Geometry: final body of the model. Coordinates: model frame, mm. A direction names the side the tool comes from. Give positions to 0.01 mm unless a question says otherwise; leave off trailing zeros. Write each loop counter-clockwise with the first axis right and the second up, starting at its lowest first coordinate (ties: lowest second). Pieces come first, ordered by that corner, then holes. Notation, with made-up numbers: (47, 66) -> (83, 66) arc R18 ccw to (83, 75) -> close; hole circle Ø8 at (-38, 39.5). An arc over 180 degrees is marked (long way). Answer in a Markdown table with one row per item. Add a question column.
Item 1: First-contact query: P1, Ø0.7, axis at y = 26, z = 2.5, coming from the +X side; P2, Ø2, axis at y = -28, z = 2, coming from the -X side; P3, Ø2, axis at y = -103.5, z = 1, coming from the -X side. Flat tips, straight axial feed; report the tip coordinate or a pass-through.
Item 2: Access query for faces 4 (the flat face through (-12.56, -102, 2)), 5 (the flat face through (5, -38.987, 2)), 6 (the flat face through (39.56, -102, 2)), 7 (the flat face through (-7, -60.137, 2)), 8 (the flat face through (2, -34.637, 2)). Directions: +Z, -Z, +X, -X, +Y, -Y. A direction counts if a zero-diameter tool reaches every point of the face in a straight line with its end or side. Return the directions, or none.
Item 3: Draft query along X for faces 1 (the flat face through (-4, -6, 2)), 2 (the flat face through (-2, -10.137, 2)), 3 (the cylindrical face through (14.54, -8.13, 1.97)). Return one class per face: +X half, -X half, draft (parallel to the pull), parting line (faces both ways), or undercut.
Item 4: Section query C-C on x = 13.5. Output: boundary loops of the cut face in (y, z), plus the area to 3 significant figures.
Item 5: Material intervals for probe 1 along Y at (x, z) = (21.5, 1); probe 2 along Y at (x, z) = (13.5, 3.1); probe 3 along X at (y, z) = (-38, 2.85), sorted ascending. Write a range as from..to.
Item 6: Section query A-A on x = -15.56. Output: boundary loops of the cut face in (y, z), plus the area to 3 significant figures.
Item 7: Section query B-B on x = 1.5. Output: boundary loops of the cut face in (y, z).
Item 8: Section query D-D on x = 42.56. Output: boundary loops of the cut face in (y, z).
```python
from build123d import *

# Parameters (mm, degrees)
SKETCH_1_R      = 2.25
SKETCH_1_R_2    = 2
SKETCH_1_R_3    = 4.1
SKETCH_1_R_4    = 1.5
EXTRUDE_1_DEPTH = 4


with BuildPart() as part:
    # 草图1 → 凸台-拉伸1 (new body)
    with BuildSketch(Plane.XY):
        with BuildLine():
            Line((0, -10.136956522), (-4, -10.136956522))
            Line((-4, -10.136956522), (-4, -2.136956522))
            Line((-4, -2.136956522), (0, -2.136956522))
            Line((0, -2.136956522), (0, 22.363043478))
            Line((0, 22.363043478), (4, 22.363043478))
            Line((4, 22.363043478), (4, 21.013043478))
            Line((4, 21.013043478), (6.6, 21.013043478))
            Line((6.6, 21.013043478), (6.6, 22.363043478))
            Line((6.6, 22.363043478), (8.6, 22.363043478))
            Line((8.6, 22.363043478), (8.6, 25.363043478))
            Line((8.6, 25.363043478), (6.6, 25.363043478))
            Line((6.6, 25.363043478), (6.6, 26.713043478))
            Line((6.6, 26.713043478), (4, 26.713043478))
            Line((4, 26.713043478), (4, 25.363043478))
            Line((4, 25.363043478), (0, 25.363043478))
            Line((0, 25.363043478), (0, 31.363043478))
            Line((0, 31.363043478), (27, 31.363043478))
            Line((27, 31.363043478), (27, 25.363043478))
            Line((27, 25.363043478), (23, 25.363043478))
            Line((23, 25.363043478), (23, 26.713043478))
            Line((23, 26.713043478), (20.4, 26.713043478))
            Line((20.4, 26.713043478), (20.4, 25.363043478))
            Line((20.4, 25.363043478), (18.4, 25.363043478))
            Line((18.4, 25.363043478), (18.4, 22.363043478))
            Line((18.4, 22.363043478), (20.4, 22.363043478))
            Line((20.4, 22.363043478), (20.4, 21.013043478))
            Line((20.4, 21.013043478), (23, 21.013043478))
            Line((23, 21.013043478), (23, 22.363043478))
            Line((23, 22.363043478), (27, 22.363043478))
            Line((27, 22.363043478), (27, -2.136956522))
            Line((27, -2.136956522), (31, -2.136956522))
            Line((31, -2.136956522), (31, -10.136956522))
            Line((31, -10.136956522), (27, -10.136956522))
            Line((27, -10.136956522), (27, -34.636956522))
            Line((27, -34.636956522), (23, -34.636956522))
            Line((23, -34.636956522), (23, -33.286956522))
            Line((23, -33.286956522), (20.4, -33.286956522))
            Line((20.4, -33.286956522), (20.4, -34.636956522))
            Line((20.4, -34.636956522), (18.4, -34.636956522))
            Line((18.4, -34.636956522), (18.4, -37.636956522))
            Line((18.4, -37.636956522), (20.4, -37.636956522))
            Line((20.4, -37.636956522), (20.4, -38.986956522))
            Line((20.4, -38.986956522), (23, -38.986956522))
            Line((23, -38.986956522), (23, -37.636956522))
            Line((23, -37.636956522), (27, -37.636956522))
            Line((27, -37.636956522), (27, -55.136956522))
            ThreePointArc((27, -55.136956522), (28.464466094, -58.672490428), (32, -60.136956522))
            Line((32, -60.136956522), (36.56, -60.136956522))
            ThreePointArc((36.56, -60.136956522), (38.681320344, -61.015636178), (39.56, -63.136956522))
            Line((39.56, -63.136956522), (39.56, -79.136956522))
            Line((39.56, -79.136956522), (49.56, -79.136956522))
            Line((49.56, -79.136956522), (49.56, -94.135010438))
            Line((49.56, -94.135010438), (39.56, -94.135010438))
            Line((39.56, -94.135010438), (39.56, -109.133064354))
            ThreePointArc((39.56, -109.133064354), (38.681320344, -111.254384698), (36.56, -112.133064354))
            Line((36.56, -112.133064354), (-9.56, -112.133064354))
            ThreePointArc((-9.56, -112.133064354), (-11.681320344, -111.254384698), (-12.56, -109.133064354))
            Line((-12.56, -109.133064354), (-12.56, -95.136956522))
            Line((-12.56, -95.136956522), (-22.56, -95.136956522))
            Line((-22.56, -95.136956522), (-22.56, -79.136956522))
            Line((-22.56, -79.136956522), (-12.56, -79.136956522))
            Line((-12.56, -79.136956522), (-12.56, -63.136956522))
            ThreePointArc((-12.56, -63.136956522), (-11.681320344, -61.015636178), (-9.56, -60.136956522))
            Line((-9.56, -60.136956522), (-5, -60.136956522))
            ThreePointArc((-5, -60.136956522), (-1.464466094, -58.672490428), (0, -55.136956522))
            Line((0, -55.136956522), (0, -37.636956522))
            Line((0, -37.636956522), (4, -37.636956522))
            Line((4, -37.636956522), (4, -38.986956522))
            Line((4, -38.986956522), (6.6, -38.986956522))
            Line((6.6, -38.986956522), (6.6, -37.636956522))
            Line((6.6, -37.636956522), (8.6, -37.636956522))
            Line((8.6, -37.636956522), (8.6, -34.636956522))
            Line((8.6, -34.636956522), (6.6, -34.636956522))
            Line((6.6, -34.636956522), (6.6, -33.286956522))
            Line((6.6, -33.286956522), (4, -33.286956522))
            Line((4, -33.286956522), (4, -34.636956522))
            Line((4, -34.636956522), (0, -34.636956522))
            Line((0, -34.636956522), (0, -10.136956522))
        make_face()
        with Locations((13.5, -6.136956522)):
            Circle(SKETCH_1_R, mode=Mode.SUBTRACT)
        with Locations((-6.5, -66.136956522)):
            Circle(SKETCH_1_R_2, mode=Mode.SUBTRACT)
        with Locations((-7.057994831, -106.133064354)):
            Circle(SKETCH_1_R_2, mode=Mode.SUBTRACT)
        with Locations((32.942005169, -106.133064354)):
            Circle(SKETCH_1_R_2, mode=Mode.SUBTRACT)
        with Locations((33.5, -66.136956522)):
            Circle(SKETCH_1_R_2, mode=Mode.SUBTRACT)
        with Locations((13.5, -66.136956522)):
            Circle(SKETCH_1_R_3, mode=Mode.SUBTRACT)
        with Locations((-15.56, -86.135010438)):
            Circle(SKETCH_1_R_4, mode=Mode.SUBTRACT)
        with Locations((42.56, -86.135010438)):
            Circle(SKETCH_1_R_4, mode=Mode.SUBTRACT)
    extrude(amount=EXTRUDE_1_DEPTH)


solid = part.part
```
Findings below:
| question | item | result |
|---|---|---|
| 1 | P1 | stops at x = 27 |
| 1 | P2 | stops at x = 0 |
| 1 | P3 | stops at x = -12.56 |
| 2 | face 4 | +Z, -Z, -X, -Y |
| 2 | face 5 | +Z, -Z |
| 2 | face 6 | +Z, -Z, +X, -Y |
| 2 | face 7 | +Z, -Z, -X, +Y |
| 2 | face 8 | +Z, -Z, -X |
| 3 | face 1 | -X half |
| 3 | face 2 | draft |
| 3 | face 3 | undercut |
| 4 | outline | (-112.13, 0) -> (-70.24, 0) -> (-70.24, 4) -> (-112.13, 4) -> close; (-62.04, 0) -> (-8.39, 0) -> (-8.39, 4) -> (-62.04, 4) -> close; (-3.89, 0) -> (31.36, 0) -> (31.36, 4) -> (-3.89, 4) -> close |
| 4 | area | 523 mm^2 |
| 5 | probe 1 | y = -112.13..-38.99, -33.29..21.01, 26.71..31.36 |
| 5 | probe 2 | y = -112.13..-70.24, -62.04..-8.39, -3.89..31.36 |
| 5 | probe 3 | x = 0..4, 6.6..20.4, 23..27 |
| 6 | outline | (-95.14, 0) -> (-87.64, 0) -> (-87.64, 4) -> (-95.14, 4) -> close; (-84.64, 0) -> (-79.14, 0) -> (-79.14, 4) -> (-84.64, 4) -> close |
| 6 | area | 52.0 mm^2 |
| 7 | outline | (-112.13, 0) -> (-37.64, 0) -> (-37.64, 4) -> (-112.13, 4) -> close; (-34.64, 0) -> (22.36, 0) -> (22.36, 4) -> (-34.64, 4) -> close; (25.36, 0) -> (31.36, 0) -> (31.36, 4) -> (25.36, 4) -> close |
| 8 | outline | (-94.14, 0) -> (-87.64, 0) -> (-87.64, 4) -> (-94.14, 4) -> close; (-84.64, 0) -> (-79.14, 0) -> (-79.14, 4) -> (-84.64, 4) -> close |
